Check sheet for the modelled part. Datum: model origin and axes. Units: mm. A direction names the side the tool comes from. Round coordinates to 2 decimals unless told otherwise and drop trailing zeros. Order: outer loops, then holes, each group sorted by start corner. A loop starts at its lowest first (then second) coordinate and runs counter-clockwise, first axis right, second up.
Q1. Cross-section at A-A on x = 14.5. Record the cut outline in (y, z), then the cut area to 3 significant figures.
Q2. Cross-section at B-B on y = 22.5. Record the cut outline in (x, z), then the cut area to 3 significant figures.
Q3. Mould release check, pull along Y, two halves, no side actions. Record for faces 1 (the flat face through (5.57, -0.15, 0.04)), 2 (the flat face through (1.394, -6.478, 0.035)), 3 (the flat face through (-5, 23, 0)): +Y half, -Y half, draft (parallel to the pull), parting line (faces both ways), or undercut.
Q4. Cross-section at C-C on z = -0.35. Record the cut outline in (x, y), then the cut area to 3 significant figures.
Q5. Set-up check for faces 4 (the flat face through (5, 22, 0)), 5 (the flat face through (-6.533, -4, 0)), 6 (the flat face through (6.533, -5, 0)), 7 (the flat face through (2.75, -9, 0)): record each of +Z, -Z, +X, -X, +Y, -Y from which the full face is reachable in a straight line by a thin tool's end or side.
Q6. Scan lines: probe 1 along X at (y, z) = (-2, -0.3); probe 2 along X at (y, z) = (42.5, 1.05); probe 3 along Y at (x, z) = (16.25, -0.4). Record each from-to range of solid material in increasing order.
Q7. Depth check by flat-ended pin: P1, Ø1.5, axis at y = -6, z = 0, coming from the +X side; P2, Ø1.5, axis at y = 18, z = -0.5, coming from the -X side; P3, Ø1, axis at y = 20.5, z = 0.5, coming from the +X side. Enter the tip coordinate at first touch or a pass-through.
from build123d import *

# Parameters (mm, degrees)
F0_W     = 10
F0_H     = 5
F4_DEPTH = 5
F6_DEPTH = 5
F7_R     = 1
F8_R     = 1


with BuildPart() as f2:
    # F2: sweep along a path in F1
    with BuildLine(Plane.XY) as f2_path:
        Line((0, 0), (0, 45))
        ThreePointArc((0, 45), (1.4644660941, 48.5355339059), (5, 50))
        Line((5, 50), (20, 50))
    # F0 (on Front) → F2 (sweep)
    with BuildSketch(Plane.XZ):
        Rectangle(F0_W, F0_H)
    sweep(path=f2_path.line)

    # F3 (on face) → F4 (join, through all)
    with BuildSketch(Plane.XY.offset(2.5)):
        Polygon((0, -12.0238676125), (6.5331561742, -8.2519481366), (6.5331561742, -0.708109185), (0, 3.0638102908), (-6.5331561742, -0.708109185), (-6.5331561742, -8.2519481366), align=None)
    extrude(amount=-F4_DEPTH)

    # F5 (on face) → F6 (cut, through all)
    with BuildSketch(Plane.XY.offset(2.5)):
        Polygon((0, -12.0238676125), (2.75, -10.4361543722), (2.75, -7.2607278916), (0, -5.6730146514), (-2.75, -7.2607278916), (-2.75, -10.4361543722), align=None)
    extrude(amount=-F6_DEPTH, mode=Mode.SUBTRACT)

    # F7
    f7_edges = [f2.edges().sort_by_distance(p)[0] for p in [
        (20, 55, 0),
        (20, 45, 0),
        (5, 45, 0),
    ]]
    fillet(f7_edges, radius=F7_R)

    # F8
    f8_edges = [f2.edges().sort_by_distance(p)[0] for p in [
        (20, 50, 2.5),
        (20, 50, -2.5),
    ]]
    fillet(f8_edges, radius=F8_R)


solid = f2.part
Results found:
1. outline: (45, -1.5) arc R1 ccw to (46, -2.5) - (54, -2.5) arc R1 ccw to (55, -1.5) - (55, 1.5) arc R1 ccw to (54, 2.5) - (46, 2.5) arc R1 ccw to (45, 1.5) - close
1. area: 49.1 mm2
2. outline: (-5, -1.5) arc R1 ccw to (-4, -2.5) - (4, -2.5) arc R1 ccw to (5, -1.5) - (5, 1.5) arc R1 ccw to (4, 2.5) - (-4, 2.5) arc R1 ccw to (-5, 1.5) - close
2. area: 49.1 mm2
3. face 1: undercut
3. face 2: -Y half
3. face 3: draft
4. outline: (-6.53, -8.25) - (-2.75, -10.44) - (-2.75, -7.26) - (0, -5.67) - (2.75, -7.26) - (2.75, -10.44) - (6.53, -8.25) - (6.53, -0.71) - (5, 0.18) - (5, 44) arc R1 cw to (6, 45) - (19, 45) arc R1 ccw to (20, 46) - (20, 54) arc R1 ccw to (19, 55) - (5, 55) arc R10 ccw to (-5, 45) - (-5, 0.18) - (-6.53, -0.71) - close
4. area: 784 mm2
5. face 4: +Z, -Z, +X
5. face 5: +Z, -Z, -X, +Y, -Y
5. face 6: +Z, -Z, +X, -Y
5. face 7: +Z, -Z, -Y
6. probe 1: x = -6.53 to 6.53
6. probe 2: x = -5 to 5
6. probe 3: y = 45 to 55
7. P1: stops at x = 6.53
7. P2: stops at x = -5
7. P3: stops at x = 5
